Can you work these out from the model? Positions are in its coordinate system, mm. A direction names the side the tool comes from. Give positions to 0.01 mm unless a question says otherwise; leave off trailing zeros. Write each loop counter-clockwise with the first axis right and the second up, starting at its lowest first coordinate (ties: lowest second). Pieces come first, ordered by that corner, then holes. Notation, with made-up numbers: (65, 88) -> (72, 88) arc R20 cw to (72, 109) -> close; hole circle Ø11 at (-25.75, 26). An arc over 180 degrees is marked (long way). One line per item, written item: value.
from build123d import *

# Parameters (mm, degrees)
BOSS_EXTRUDE1_DEPTH     = 30
CUT_EXTRUDE1_DEPTH      = 79.102496759
CUT_EXTRUDE1_DEPTH_BACK = 79.102496759
SKETCH2_W               = 11
SKETCH2_H               = 60
SKETCH3_W               = 40
SKETCH3_H               = 10
CUT_EXTRUDE2_DEPTH      = 20
FILLET2_R               = 3
FILLET3_R               = 20
CUT_EXTRUDE3_DEPTH      = 71.710678119
CUT_EXTRUDE3_DEPTH_BACK = 71.710678119
SKETCH4_R               = 2
CUT_EXTRUDE4_DEPTH      = 71.710678119
CUT_EXTRUDE4_DEPTH_BACK = 71.710678119
SKETCH5_R               = 2
FILLET4_R               = 2


with BuildPart() as part:
    # Sketch1 → Boss-Extrude1 (new body)
    with BuildSketch(Plane.XY):
        Polygon((0, 0), (-40, 0), (-40, 40), (-50, 40), (-50, -10), (10, -10), (10, 40), (0, 40), align=None)
    extrude(amount=BOSS_EXTRUDE1_DEPTH)

    # Sketch2 → Cut-Extrude1 (cut, two sides: drawn at the far end of the back side and taken through both)
    with BuildSketch(Plane(origin=(10, 0, 0), x_dir=(0, 0, -1), z_dir=(1, 0, 0)).offset(-CUT_EXTRUDE1_DEPTH_BACK)):
        with Locations((-15, 40)):
            Rectangle(SKETCH2_W, SKETCH2_H)
    extrude(amount=CUT_EXTRUDE1_DEPTH + CUT_EXTRUDE1_DEPTH_BACK, mode=Mode.SUBTRACT)

    # Sketch3 → Cut-Extrude2 (cut)
    with BuildSketch(Plane(origin=(0, 0, 0), x_dir=(-1, 0, 0), z_dir=(0, 0, -1))):
        with Locations((20, -5)):
            Rectangle(SKETCH3_W, SKETCH3_H)
    extrude(amount=-CUT_EXTRUDE2_DEPTH, mode=Mode.SUBTRACT)

    # Fillet2
    fillet2_edges = [part.edges().sort_by_distance(p)[0] for p in [
        (-20, -10, 30),
        (-20, 0, 20),
        (-20, -10, 20),
        (-20, 0, 30),
    ]]
    fillet(fillet2_edges, radius=FILLET2_R)

    # Fillet3
    fillet3_edges = [part.edges().sort_by_distance(p)[0] for p in [
        (5, -10, 0),
        (-45, -10, 0),
    ]]
    fillet(fillet3_edges, radius=FILLET3_R)

    # Sketch4 → Cut-Extrude3 (cut, two sides: drawn at the far end of the back side and taken through both)
    with BuildSketch(Plane(origin=(0, 0, 0), x_dir=(-1, 0, 0), z_dir=(0, 0, -1)).offset(-CUT_EXTRUDE3_DEPTH_BACK)):
        with Locations((-5, 35)):
            Circle(SKETCH4_R)
    extrude(amount=CUT_EXTRUDE3_DEPTH + CUT_EXTRUDE3_DEPTH_BACK, mode=Mode.SUBTRACT)

    # Sketch5 → Cut-Extrude4 (cut, two sides: drawn at the far end of the back side and taken through both)
    with BuildSketch(Plane(origin=(0, 0, 0), x_dir=(-1, 0, 0), z_dir=(0, 0, -1)).offset(-CUT_EXTRUDE4_DEPTH_BACK)):
        with Locations((45, 35)):
            Circle(SKETCH5_R)
    extrude(amount=CUT_EXTRUDE4_DEPTH + CUT_EXTRUDE4_DEPTH_BACK, mode=Mode.SUBTRACT)

    # Fillet4
    fillet4_edges = [part.edges().sort_by_distance(p)[0] for p in [
        (-45, 40, 30),
        (5, 40, 30),
        (5, 40, 0),
        (-45, 40, 0),
    ]]
    fillet(fillet4_edges, radius=FILLET4_R)


solid = part.part
1) If we section it at A-A (x = -45): Write out the boundary of the cut face in (y, z), and give its area (3 significant figures).
Answer list:
outline: (-10, 20) arc R20 ccw to (10, 0) -> (33, 0) -> (33, 9.5) -> (10, 9.5) -> (10, 20.5) -> (33, 20.5) -> (33, 30) -> (-7, 30) arc R3 ccw to (-10, 27) -> close; (37, 0) -> (38, 0) arc R2 ccw to (40, 2) -> (40, 9.5) -> (37, 9.5) -> close; (37, 20.5) -> (40, 20.5) -> (40, 28) arc R2 ccw to (38, 30) -> (37, 30) -> close
area: 1,000 mm^2
2) We'd pull the mould along Y, two halves only. Please class faces 4 (the face through (5, 25, 20.5)), 5 (the face through (5, 33, 5)), 6 (the face through (-44.93, -4.297, 6.014)), 7 (the face through (5, 10, 15)): released by +Y, released by -Y, zero draft, split by the parting line, or undercut.
Answer list:
face 4: zero draft
face 5: undercut
face 6: released by -Y
face 7: released by +Y
3) If we section it at D-D (y = 9): Write out the boundary of the cut face in (x, z).
Answer list:
outline: (-50, 0.03) -> (-40, 0.03) -> (-40, 30) -> (-50, 30) -> close; (0, 0.03) -> (10, 0.03) -> (10, 30) -> (0, 30) -> close
4) For faces 1 (the face through (-45, 25, 20.5)), 2 (the face through (-20, -5, 20)), 3 (the face through (4.93, 39.4, 0.57)), which set-ups out of +Z, -Z, +X, -X, +Y, -Y let a thin tool reach every point of the face, with its end or its side?
Answer list:
face 1: +X, -X, +Y
face 2: -Z, +Y, -Y
face 3: -Z, +X, -X, +Y
5) I need wall thicknesses on L1, parallel to X at y = 35, z = 2.75; L2, parallel to Y at x = -45, z = 23.5; L3, parallel to X at y = 20.5, z = 23. Which ranges of each line are inside material? Lowest first, please.
Answer list:
L1: x = -50 to -47, -43 to -40, 0 to 3, 7 to 10
L2: y = -10 to 33, 37 to 40
L3: x = -50 to -40, 0 to 10
6) If we section it at C-C (z = 6.5): Write out the boundary of the cut face in (x, y), and give its area (3 significant figures).
Answer list:
outline: (-50, -4.76) -> (-40, -4.76) -> (-40, 40) -> (-50, 40) -> close; (0, -4.76) -> (10, -4.76) -> (10, 40) -> (0, 40) -> close; hole circle Ø4 at (-45, 35); hole circle Ø4 at (5, 35)
area: 870 mm^2
7) If we section it at B-B (y = 31.5): Write out the boundary of the cut face in (x, z), and give its area (3 significant figures).
Answer list:
outline: (-50, 0) -> (-40, 0) -> (-40, 9.5) -> (-50, 9.5) -> close; (-50, 20.5) -> (-40, 20.5) -> (-40, 30) -> (-50, 30) -> close; (0, 0) -> (10, 0) -> (10, 9.5) -> (0, 9.5) -> close; (0, 20.5) -> (10, 20.5) -> (10, 30) -> (0, 30) -> close
area: 380 mm^2
8) Will these pins go through, and if not, where does the flat tip stop? pin 1 (2 mm diameter, centred on y = 12.5, z = 14, fed in from +X); pin 2 (5 mm diameter, centred on x = 5, z = 17.5, fed in from +Y); pin 3 (1.2 mm diameter, centred on x = -27.5, y = -4.5, fed in from -Z); pin 4 (1.2 mm diameter, centred on x = -20.5, z = 24.5, fed in from +Y).
Answer list:
pin 1: passes through
pin 2: stops at y = 10
pin 3: stops at z = 20
pin 4: stops at y = 0
